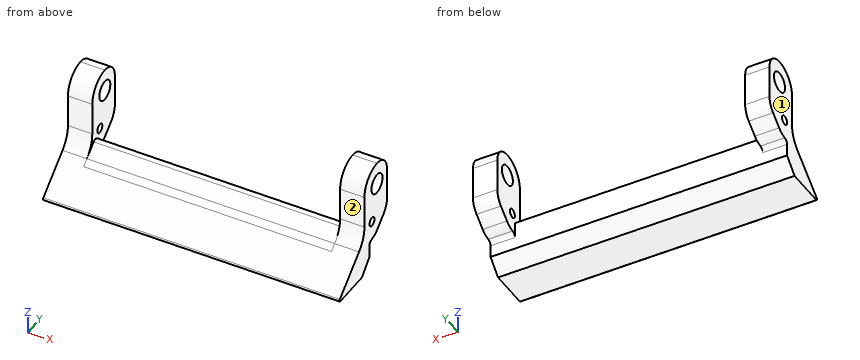
Autodesk Inventor part; units mm, degrees
ref_plane "YZ Plane" through (0, 0, 0) normal (1, 0, 0) x (0, 1, 0)
ref_plane "XZ Plane" through (0, 0, 0) normal (0, 1, 0) x (-1, 0, 0)
ref_plane "XY Plane" through (0, 0, 0) normal (0, 0, 1) x (1, 0, 0)
sketch "Skizze1" plane through (0, 0, 0) normal (1, 0, 0) x (0, 1, 0)
  line L0 (-4.1616, 7.0772) -> (-12, 0.5)
  line L1 (-12, 0) -> (-3, 0)
  line L2 (-12, 0.5) -> (-12, 0)
  line L3 (0, 5) -> (8, 11.7128)
  circle A0 centre (3, 19) radius 0.5
  line L4 (-2, 11.7128) -> (-2, 24)
  line L5 (-2, 24) -> (8, 24)
  line L6 (8, 24) -> (8, 11.7128)
  line L7 (0, 3) -> (-3, 0)
  line L8 (8, 11.7128) -> (-2, 11.7128) construction
  arc A1 (-4.1616, 7.0772) -> (-2, 11.7128) centre (-8.0514, 11.7128) ccw
  line L9 (0, 5) -> (0, 3)
  line L10 (3, 19) -> (3, 0) construction
  point P0 (0, 0)
  dimension "d40" = 0.5
  dimension "d44" = 1
  dimension "d59" = 10
  dimension "d60" = 45
  dimension "d61" = 5
  dimension "d63" = 40
  dimension "d78" = 3
  dimension "d79" = 12
  dimension "d80" = 0
  dimension "d81" = 19
  dimension "d82" = 5
  dimension "d83" = 3
extrude "Extrusion1" add sketch "Skizze1" along normal mid plane 67
sketch "Skizze6" plane through (0, 0, 0) normal (0, 1, 0) x (-1, 0, 0)
  line L0 (33.5, 0.5) -> (-33.5, 0.5)
  line L1 (-33.5, 7.0772) -> (-33.5, 0.5)
  line L2 (33.5, 0.5) -> (33.5, 7.0772)
  line L3 (-27.5, 6) -> (27.5, 6)
  line L4 (27.5, 6) -> (27.5, 31)
  line L5 (27.5, 31) -> (-27.5, 31)
  line L6 (-27.5, 31) -> (-27.5, 6)
  line L7 (0, -6.2) -> (0, 37.2)
  line L8 (33.5, 0) -> (-33.5, 0)
  line L9 (-33.5, 0) -> (33.5, 0)
  point P0 (0, 0)
  point P1 (-33, 10)
  point P2 (33, 10)
  dimension "d45" = 6
  dimension "d46" = 25
  dimension "d50" = 6
extrude "Extrusion4" cut sketch "Skizze6" along normal mid plane 16
sketch "Skizze3" plane through (-33.5, 0, 0) normal (-1, 0, 0) x (0, 0, 1)
  line L0 (0, -3) -> (0, -12)
  line L1 (0.5, -12) -> (7.0772, -4.1616)
  line L2 (0, -12) -> (0, 0) construction
  line L3 (0, 12) -> (0, -16)
  line L4 (0, -12) -> (0.5, -12)
  line L5 (11.7128, 8) -> (5, 0)
  line L6 (11.7128, -2) -> (24, -2)
  line L7 (24, -2) -> (24, 8)
  line L8 (24, 8) -> (11.7128, 8)
  circle A0 centre (19, 3) radius 0.5
  line L9 (3, 0) -> (0, -3)
  arc A1 (11.7128, -2) -> (7.0772, -4.1616) centre (11.7128, -8.0514) ccw
  line L10 (5, 0) -> (3, 0)
hole "Bohrung1" at (-33.5, 3, 19) direction (1, 0, 0) diameter 4.4 end through all
sketch "Skizze4" plane through (-33.5, 0, 0) normal (-1, 0, 0) x (0, 0, 1)
  line L0 (0, 12) -> (0, -16)
  line L1 (-5.8, 0) -> (34.8, 0)
  point P0 (29, 0)
  point P1 (11, 1)
  dimension "d38" = 11
  dimension "d84" = 1
hole "Bohrung2" at (-33.5, 1, 11) direction (1, 0, 0) diameter 2 end through all
fillet "Rundung2" radius 5 6 edges at (30.5, -2, 24) (30.5, 8, 24) (-30.5, 8, 24) (-30.5, -2, 24) (30.5, 8, 11.7128) (-30.5, 8, 11.7128)
fillet "Rundung8" radius 0.36 2 edges at (0, -12, 0.5) (0, -12, 0)
sketch "Skizze7" plane through (-27.5, 1.1918, 6) normal (0, 0, 1) x (1, 0, 0)
  line L0 (0, 0) -> (55, 0)
  line L1 (0, 0) -> (0, -6.6371)
  line L2 (55, -6.6371) -> (0, -6.6371)
  line L3 (55, -6.6371) -> (55, 0)
  line L4 (-19.4, -1.1918) -> (74.4, -1.1918)
  point P0 (27.5, -1.1918)
  point P1 (0, -1.1918)
  point P2 (55, -1.1918)
extrude "Extrusion5" cut sketch "Skizze7" against normal through all contours L0 L3 L4 L1
sketch "Skizze8" plane through (-27.5, -5.4454, 6) normal (1, 0, 0) x (0, 0, -1)
  line L0 (-8.0443, 13.4454) -> (-13, 13.4454)
  line L1 (-10.5222, 13.4454) -> (-10.5222, 12.4454)
  line L2 (-10.5222, 12.4454) -> (-17.4656, 12.4454)
  line L3 (-17.4656, 12.4454) -> (-4.9838, 12.4454)
  line L4 (-4.9838, 12.4454) -> (-4.9838, 14.4351)
  line L5 (-4.9838, 14.4351) -> (-17.4656, 14.4351)
  line L6 (-17.4656, 14.4351) -> (-17.4656, 12.4454)
  point P0 (6, 5.4454)
  dimension "d90" = 1
extrude "Extrusion6" cut sketch "Skizze8" along normal mid plane 200
fillet "Rundung10" radius 4 4 edges at (30.5, 7, 11.0443) (30.5, 7, 22.0001) (-30.5, 7, 22.0001) (-30.5, 7, 11.0443)
sketch "Skizze9" plane through (-27.5, -2, 19) normal (1, 0, 0) x (0, 0, -1)
  line L0 (9.3252, 7.5712) -> (14, 2)
  line L1 (14, 2) -> (14, 3)
  line L2 (14, 3) -> (12.8, 3)
  line L3 (12.8, 3) -> (14, 3)
  line L4 (14, 3) -> (14, 4.2192)
  line L5 (14, 4.2192) -> (12.8, 4.2192)
  line L6 (12.8, 4.2192) -> (12.8, 3)
  line L7 (12.3, 4.7192) -> (14.5, 4.7192)
  line L8 (14.5, 4.7192) -> (14.5, 2.5)
  line L9 (14.5, 2.5) -> (12.3, 2.5)
  line L10 (12.3, 2.5) -> (12.3, 4.7192)
  line L11 (12.3, 2.5) -> (12.3, 1.2569)
  line L12 (12.3, 1.2569) -> (14.6235, 1.2569)
  line L13 (12.3, 1.2569) -> (11.55, 1.2569)
  line L14 (11.55, 1.2569) -> (11.55, 4.7192)
  line L15 (11.55, 4.7192) -> (12.3, 4.7192)
  point P0 (19, 2)
  point P1 (13.5805, 2.5)
  point P2 (12.3, 4.026)
  point P3 (11.55, 4.45)
  point P4 (13.1609, 3)
  point P5 (14, 2.5)
  dimension "d95" = 1
  dimension "d96" = 1.2
  dimension "d97" = 0.5
  dimension "d103" = 0.75
extrude "Extrusion7" cut sketch "Skizze9" along normal mid plane 200 contours L10 L7 L8 L9 L1 L4 L5 L6 L0 | L0 L6 L2 L9 L10 | L6 L5 L4 L2 L0 | L0 L2 L6 | L2 L1 L9 L0 | L9 L1 L0
fillet "Rundung12" radius 4 2 edges at (30.5, 2.026, 6.7) (-30.5, 2.026, 6.7)
sketch "Skizze16" plane through (-27.5, 0, 6) normal (0, 0, 1) x (1, 0, 0)
  line L0 (27.5, 0) -> (27.5, -5.4454)
  line L1 (55, -5.4454) -> (0, -5.4454)
  line L2 (27.5, -5.4454) -> (27.5, -26.9454)
  circle A0 centre (27.5, -26.9454) radius 21.5
  circle A1 centre (27.5, -26.9454) radius 24.5
  line L3 (0, -5.4454) -> (0, 0)
  line L4 (-6, 0) -> (61, 0)
  line L5 (0, 0) -> (55, 0)
  line L6 (55, 0) -> (55, -5.4454)
  line L7 (55, -5.4454) -> (0, -5.4454)
  line L8 (0, -5.4454) -> (0, 0)
  point P0 (15.7527, -5.4454)
  point P1 (39.2473, -5.4454)
  point P2 (55, 0)
  dimension "d122" = 21.5
  dimension "d123" = 3
extrude "Extrusion11" add sketch "Skizze16" along normal blind 5 contours L4 L6 L1 A1 L0 | L0 A1 L1 L3 L4 | A1 L1 L0 | L0 L1 A1
sketch "Skizze18" plane through (27.5, -5.4454, 11) normal (1, 0, 0) x (0, 0, -1)
  line L0 (10.3642, -6.3928) -> (3.9228, 1.2837)
  line L1 (10.3642, -6.3928) -> (0, 5.9588)
  line L2 (0, 0) -> (0, 3.4032)
  line L3 (0, 5.9588) -> (0, 0)
  line L4 (0, 0) -> (5, 0)
  point P0 (11, 5.4454)
  point P1 (5, 0)
extrude "Extrusion12" cut sketch "Skizze18" against normal up to surface (55 mm away)
sketch "Skizze19" plane through (27.5, -2, 11.7128) normal (-1, 0, 0) x (0, 0, 1)
  circle A0 centre (-0.7128, 3) radius 1
  circle A1 centre (-0.7128, 3) radius 2
  point P0 (-11.7128, 2)
  dimension "d131" = 4
extrude "Extrusion13" cut sketch "Skizze19" along normal up to surface (55 mm away) contours A0 | A1
sketch "Skizze22" plane through (33.5, 0, 0) normal (1, 0, 0) x (0, 0, -1)
  line L0 (0, -3) -> (-3, 0)
  line L1 (-5.4195, 0.5) -> (-6.7, 0.5)
  line L2 (-3, 0) -> (-6.7, 0)
  line L3 (-6.7, 0) -> (-6.7, 0.5)
  line L4 (-6.7, 0.5) -> (-3, 0.5)
  line L5 (-3, 0.5) -> (-3, 0)
  point P0 (0, 0)
  point P1 (-5.4195, 0.5)
extrude "Extrusion14" cut sketch "Skizze22" against normal up to surface (67 mm away)
fillet "Rundung22" radius 1 2 edges at (30.5, 0, 6.7) (-30.5, 0, 6.7)
sketch "Skizze23" plane through (-33.5, -2, 11.7128) normal (0, -1, 0) x (1, 0, 0)
  line L0 (0, 8.2872) -> (0, 12.2872)
  line L1 (0, 12.2872) -> (67, 12.2872)
  line L2 (67, 12.2872) -> (67, -11.7128)
  line L3 (67, -11.7128) -> (0, -11.7128)
  line L4 (0, -11.7128) -> (0, 12.2872)
  line L5 (66.4, 11.6872) -> (0.6, 11.6872)
  line L6 (0.6, 11.6872) -> (0.6, -11.1128)
  line L7 (0.6, -11.1128) -> (66.4, -11.1128)
  line L8 (66.4, -11.1128) -> (66.4, 11.6872)
  line L9 (66.4, 11.6872) -> (66.4, 12.2872)
  line L10 (66.4, -11.1128) -> (66.4, -11.7128)
  line L11 (0.6, -11.1128) -> (0.6, -11.7128)
  line L12 (0.6, 11.6872) -> (0.6, 12.2872)
  dimension "d146" = 0.6
extrude "Extrusion15" cut sketch "Skizze23" along normal mid plane 100 contours L0 L1 L12 L6 L11 L3 L4 | L1 L2 L3 L10 L8 L9
fillet "Rundung23" radius 1 1 edges at (0, -0.7143, 9.9698)
properties part number "Schaufel" material "Aluminium 6061"
Build history of the part. All positions in model axes, mm. Face numbers are marked on the shaded views. A direction names the side the tool comes from. Round coordinates to 2 decimals unless told otherwise and drop trailing zeros. Write each loop counter-clockwise with the first axis right and the second up, starting at its lowest first coordinate (ties: lowest second). Pieces come first, ordered by that corner, then holes. Notation, with made-up numbers: (-0.75, 82) - (42.25, 82) arc R15 cw to (42.25, 106) - close; hole circle Ø1 at (-13, -18.5). An arc over 180 degrees is marked (long way). One line per question, with ' | ' between items.
1. Band-saw the part on C-C, the plane z = 8.25. Write the cut outline in (x, y), and give its area (3 significant figures).
Results are:
outline: (-32.9, -3.09) - (-27.5, -3.09) - (-27.5, -2.76) - (27.5, -2.76) - (27.5, -3.09) - (32.9, -3.09) - (32.9, 3.87) - (27.5, 3.87) - (27.5, 0) - (-27.5, 0) - (-27.5, 3.87) - (-32.9, 3.87) - close | area: 227 mm^2
2. Drill centre lines: line 1 along Y through (x, z) = (-28.7, 19); line 2 along X through (y, z) = (1.25, 16.5); line 3 along Z through (x, y) = (29.8, 1). Where is each one in solid material? Low to high. Write a range as from..to.
Results are:
line 1: -2..0.8, 5.2..7 | line 2: -32.9..-27.5, 27.5..32.9 | line 3: 6.72..10, 12..18.08, 19.92..23.58
3. Band-saw the part on D-D, the plane z = 11. Give the number of separate pieces and of enclosed holes in the cut face, and give its area (3 significant figures).
Results are:
separate pieces: 4 | enclosed holes: 0 | area: 71.8 mm^2
4. Band-saw the part on A-A, the plane z = 18.25. Write the cut outline in (x, y).
Results are:
outline: (-32.9, -2) - (-27.5, -2) - (-27.5, 0.93) - (-32.9, 0.93) - close; (-32.9, 5.07) - (-27.5, 5.07) - (-27.5, 7) - (-32.9, 7) - close; (27.5, -2) - (32.9, -2) - (32.9, 0.93) - (27.5, 0.93) - close; (27.5, 5.07) - (32.9, 5.07) - (32.9, 7) - (27.5, 7) - close
5. Tool access for the marked faces 1 and 2: list every direction of +Z, -Z, +X, -X, +Y, -Y with a clear straight run to the whole face (end or side of a thin tool).
Results are:
face 1: +Z, -Z, -X, +Y, -Y | face 2: +Z, +X, -X, -Y
6. Drop flat-ended pins along their axis: pin 1 Ø10 at (x, y) = (-18, -9) entering from +Z; pin 2 Ø2.5 at (y, z) = (1, 11) entering from +X; pin 3 Ø1.6 at (x, z) = (-30.5, 16.5) entering from -Y; pin 4 Ø3 at (x, z) = (11.5, 7.5) entering from +Y. Give the stop position or say it passes through.
Results are:
pin 1: z = 7.21 | pin 2: x = 32.9 | pin 3: y = -2 | pin 4: y = 0
7. Band-saw the part on B-B, the plane z = 14.5. Write the cut outline in (x, y).
Results are:
outline: (-32.9, -2) - (-27.5, -2) - (-27.5, 7) - (-32.9, 7) - close; (27.5, -2) - (32.9, -2) - (32.9, 7) - (27.5, 7) - close
